```python
from build123d import *

# Parameters (mm, degrees)
SKETCH_1_W          = 20
SKETCH_1_H          = 42
EXTRUDE_1_DEPTH     = 3
SKETCH_2_W          = 20
SKETCH_2_H          = 3.5
EXTRUDE_2_DEPTH     = 47
SKETCH_3_R          = 1.5
CUT_EXTRUDE_1_DEPTH = 69.293484316
SKETCH_4_W          = 35
SKETCH_4_H          = 3
EXTRUDE_3_DEPTH     = 20
SKETCH_8_W          = 20
SKETCH_8_H          = 20
EXTRUDE_5_DEPTH     = 2
SKETCH_9_R          = 6.2
CUT_EXTRUDE_4_DEPTH = 2
CUT_EXTRUDE_4_DRAFT = -45
SKETCH_10_R         = 4.2
CUT_EXTRUDE_5_DEPTH = 3
CUT_EXTRUDE_5_DRAFT = -10
SKETCH_11_R         = 1.5
CUT_EXTRUDE_6_DEPTH = 3


with BuildPart() as part:
    # 草图1 → 凸台-拉伸1 (new body)
    with BuildSketch(Plane(origin=(0, 0, 0), x_dir=(1, 0, 0), z_dir=(0, 1, 0))):
        with Locations((10, -21)):
            Rectangle(SKETCH_1_W, SKETCH_1_H)
    extrude(amount=EXTRUDE_1_DEPTH)

    # 草图2 → 凸台-拉伸2 (add)
    with BuildSketch(Plane(origin=(0, 3, 0), x_dir=(1, 0, 0), z_dir=(0, 1, 0))):
        with Locations((10, -40.25)):
            Rectangle(SKETCH_2_W, SKETCH_2_H)
        with Locations((10, -1.75)):
            Rectangle(SKETCH_2_W, SKETCH_2_H)
    extrude(amount=EXTRUDE_2_DEPTH)

    # 草图3 → 切除-拉伸1 (cut, through all)
    with BuildSketch(Plane.XY.offset(42)):
        with Locations((10, 20)):
            Circle(SKETCH_3_R)
    extrude(amount=-CUT_EXTRUDE_1_DEPTH, mode=Mode.SUBTRACT)

    # 草图4 → 凸台-拉伸3 (add)
    with BuildSketch(Plane(origin=(20, 0, 0), x_dir=(0, 0, -1), z_dir=(1, 0, 0))):
        with Locations((-21, 48.5)):
            Rectangle(SKETCH_4_W, SKETCH_4_H)
    extrude(amount=-EXTRUDE_3_DEPTH)

    # 草图8 → 凸台-拉伸5 (add)
    with BuildSketch(Plane(origin=(0, 50, 0), x_dir=(1, 0, 0), z_dir=(0, 1, 0))):
        with Locations((10, -21)):
            Rectangle(SKETCH_8_W, SKETCH_8_H)
    extrude(amount=EXTRUDE_5_DEPTH)


with BuildPart() as cut_extrude_4_tool:
    # 草图9 → 切除-拉伸4 (with draft: the straight prism first)
    with BuildSketch(Plane(origin=(0, 52, 0), x_dir=(1, 0, 0), z_dir=(0, 1, 0))):
        with Locations((10, -21)):
            Circle(SKETCH_9_R)
    extrude(amount=-CUT_EXTRUDE_4_DEPTH)
    # 切除-拉伸4: the draft: its side faces are tilted about the plane it starts from
    cut_extrude_4_sides = [cut_extrude_4_tool.faces().sort_by_distance(p)[0] for p in [
        (3.8, 51, 21),
    ]]
    draft(cut_extrude_4_sides, Plane(origin=(0, 52, 0), x_dir=(1, 0, 0), z_dir=(0, 1, 0)), CUT_EXTRUDE_4_DRAFT)


with BuildPart() as part_1:
    add(part.part)

    # 切除-拉伸4: cut by cut_extrude_4_tool
    add(cut_extrude_4_tool.part, mode=Mode.SUBTRACT)


with BuildPart() as cut_extrude_5_tool:
    # 草图10 → 切除-拉伸5 (with draft: the straight prism first)
    with BuildSketch(Plane(origin=(0, 50, 0), x_dir=(1, 0, 0), z_dir=(0, 1, 0))):
        with Locations((10, -21)):
            Circle(SKETCH_10_R)
    extrude(amount=-CUT_EXTRUDE_5_DEPTH)
    # 切除-拉伸5: the draft: its side faces are tilted about the plane it starts from
    cut_extrude_5_sides = [cut_extrude_5_tool.faces().sort_by_distance(p)[0] for p in [
        (5.8, 48.5, 21),
    ]]
    draft(cut_extrude_5_sides, Plane(origin=(0, 50, 0), x_dir=(1, 0, 0), z_dir=(0, 1, 0)), CUT_EXTRUDE_5_DRAFT)


with BuildPart() as part_2:
    add(part_1.part)

    # 切除-拉伸5: cut by cut_extrude_5_tool
    add(cut_extrude_5_tool.part, mode=Mode.SUBTRACT)

    # 草图11 → 切除-拉伸6 (cut)
    with BuildSketch(Plane(origin=(0, 0, 0), x_dir=(-1, 0, 0), z_dir=(0, -1, 0))):
        with Locations(Location((-10, -32, 0), (0, 0, 90))):
            Circle(SKETCH_11_R)
        with Locations(Location((-10, -10, 0), (0, 0, 90))):
            Circle(SKETCH_11_R)
    extrude(amount=-CUT_EXTRUDE_6_DEPTH, mode=Mode.SUBTRACT)


solid = part_2.part
```
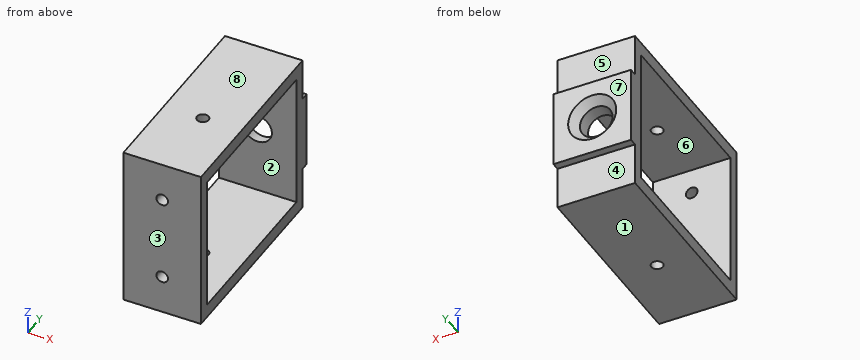
Work out the finished part from the listing and answer in its coordinate system (mm). Face numbers are marked on the shaded views. A direction names the side the tool comes from. Round coordinates to 2 decimals unless told otherwise and drop trailing zeros. Loops run counter-clockwise (first coordinate to the right, second up) from the corner with the lowest first, then second, coordinate; pieces in that order, holes last.
(1) Each of these flat-tipped pins is pushed along its axis until it touches: P1, Ø12, axis at x = 11, z = 6, coming from the -Y side; P2, Ø3.5, axis at x = 13.5, z = 6.5, coming from the +Y side; P3, Ø1.6, axis at x = 6.5, y = 51, coming from the -Z side. Where does it stop, or does it pass through?
Computed values:
P1: stops at y = 0
P2: stops at y = 50
P3: stops at z = 11
(2) The mould has two halves that part along Z. Classify the marked faces 6, 7 and 8: pulls with the +Z half, pulls with the -Z half, needs draft (parallel to the pull), parting line crosses it, or undercut.
Computed values:
face 6: undercut
face 7: needs draft
face 8: pulls with the +Z half
(3) The part is cut by section B-B, the plane z = 35. Give the vertices of the cut face in (x, y), and give its area (3 significant figures).
Computed values:
outline: (0, 0) - (20, 0) - (20, 3) - (0, 3) - close; (0, 47) - (20, 47) - (20, 50) - (0, 50) - close
area: 120 mm2
(4) The part is cut by section A-A, the plane y = 20. Give the vertices of the cut face in (x, z).
Computed values:
outline: (0, 0) - (8.5, 0) - (8.5, 3.5) - (0, 3.5) - close; (0, 38.5) - (8.5, 38.5) - (8.5, 42) - (0, 42) - close; (11.5, 0) - (20, 0) - (20, 3.5) - (11.5, 3.5) - close; (11.5, 38.5) - (20, 38.5) - (20, 42) - (11.5, 42) - close
(5) For the marked faces 1, 2, 3, 4 and 5, determine the directions among +Z, -Z, +X, -X, +Y, -Y from which every point of the face is accessible in a straight line to the end or side of a thin tool.
Computed values:
face 1: -Z, +X, -X, +Y, -Y
face 2: +X, -X
face 3: +Z, -Z, +X, -X, -Y
face 4: -Z, +X, -X, +Y
face 5: +Z, +X, -X, +Y
(6) The part is cut by section D-D, the plane z = 10. Give the vertices of the cut face in (x, y), and give its area (3 significant figures).
Computed values:
outline: (0, 0) - (8.5, 0) - (8.5, 3) - (0, 3) - close; (0, 47) - (20, 47) - (20, 50) - (0, 50) - close; (11.5, 0) - (20, 0) - (20, 3) - (11.5, 3) - close
area: 111 mm2
(7) The part is cut by section C-C, the plane x = 17.75. Give the vertices of the cut face in (y, z).
Computed values:
outline: (0, 0) - (50, 0) - (50, 11) - (52, 11) - (52, 31) - (50, 31) - (50, 42) - (0, 42) - close; hole (3, 3.5) - (47, 3.5) - (47, 38.5) - (3, 38.5) - close
(8) Find the intervals of material crossed by L1, parallel to Z at x = 15, y = 29; L2, parallel to Y at x = 7.5, z = 28.5; L3, parallel to Y at x = 10, z = 40.05, in increasing order.
Computed values:
L1: z = 0 to 3.5, 38.5 to 42
L2: y = 0 to 3, 47 to 52
L3: y = 0 to 18.5, 21.5 to 50
